from build123d import *

# Parameters (mm, degrees)
SKETCH1_R           = 5
BOSS_EXTRUDE1_DEPTH = 47.5
SKETCH2_W           = 1.5
SKETCH2_H           = 0.94


with BuildPart() as part:
    # Sketch1 → Boss-Extrude1 (new, symmetric)
    with BuildSketch(Plane.XY):
        Circle(SKETCH1_R)
    extrude(amount=BOSS_EXTRUDE1_DEPTH, both=True)

    # Sketch2 → Cut-Revolve1 (revolve, cut)
    with BuildSketch(Plane(origin=(0, 0, 0), x_dir=(1, 0, 0), z_dir=(0, 1, 0))):
        with Locations((-4.25, 38.03)):
            Rectangle(SKETCH2_W, SKETCH2_H)
    revolve(axis=Axis((0, 0, -47.5), (0, 0, 1)), mode=Mode.SUBTRACT)


solid = part.part
Read the model definition and answer for the solid it produces. Units are mm, in the model's axes. A direction names the side the tool comes from. Round coordinates to 2 decimals unless told otherwise and drop trailing zeros. Loops run counter-clockwise (first coordinate to the right, second up) from the corner with the lowest first, then second, coordinate; pieces in that order, holes last.
Q1. Which of the six approach directions +Z, -Z, +X, -X, +Y, -Y give full straight-line access (tool end or side, diameter ignored) to faces 1 (the face through (-3.233, 1.341, -38.037)), 2 (the face through (-1.08, -4.88, 5.57))?
Q2. Consider probe 1 along Z at (x, y) = (-3.5, 1); probe 2 along X at (y, z) = (-0.25, 37); probe 3 along X at (y, z) = (4.5, -37.5). Determine where each line is inside the solid, lowest interval first.
Q3. Section B-B on z = -36 is taken. Write down the section's boundary in (x, y).
Q4. Each of these flat-tipped pins is pushed along its axis until it touches: pin 1 (1.5 mm diameter, centred on x = -3.5, z = 23, fed in from +Y); pin 2 (1 mm diameter, centred on y = -4, z = 29.5, fed in from +X); pin 3 (1 mm diameter, centred on x = 3.5, z = 16.5, fed in from -Y). Where does it stop, or does it pass through?
Q5. Determine the mould class of faces 3 (the face through (-2.2, 3.3, -37.56)), 4 (the face through (0, 0, -47.5)), 5 (the face through (-1.08, -4.88, -42.94)), 6 (the face through (0, 0, 47.5)) for opening direction Z: released by +Z, released by -Z, zero draft, split by the parting line, or undercut.
Q6. Section A-A on y = -1.75 is taken. Write down the section's boundary in (x, z).
Output:
1. face 1: none
1. face 2: +Z, -Z
2. probe 1: z = -47.5 to -38.5, -37.56 to 47.5
2. probe 2: x = -4.99 to 4.99
2. probe 3: x = -2.18 to 2.18
3. outline: circle Ø10 at (0, 0)
4. pin 1: stops at y = 4.18
4. pin 2: stops at x = 3.57
4. pin 3: stops at y = -4
5. face 3: undercut
5. face 4: released by -Z
5. face 5: zero draft
5. face 6: released by +Z
6. outline: (-4.68, -47.5) - (4.68, -47.5) - (4.68, -38.5) - (3.03, -38.5) - (3.03, -37.56) - (4.68, -37.56) - (4.68, 47.5) - (-4.68, 47.5) - (-4.68, -37.56) - (-3.03, -37.56) - (-3.03, -38.5) - (-4.68, -38.5) - close
